Source: CAD feature listing. Evaluate the final solid. Frame: model axes, mm. Give positions to 0.01 mm unless a question says otherwise; leave off trailing zeros. Loops run counter-clockwise (first coordinate to the right, second up) from the corner with the lowest first, then second, coordinate; pieces in that order, holes last. Notation, with made-up numbers: M 14.25,13.25 L 55.25,13.25 A36 ccw 55.25,50.25 Z; hole C 3,72 d2. An arc over 180 degrees is marked long. Answer in a Markdown table with one row per item.
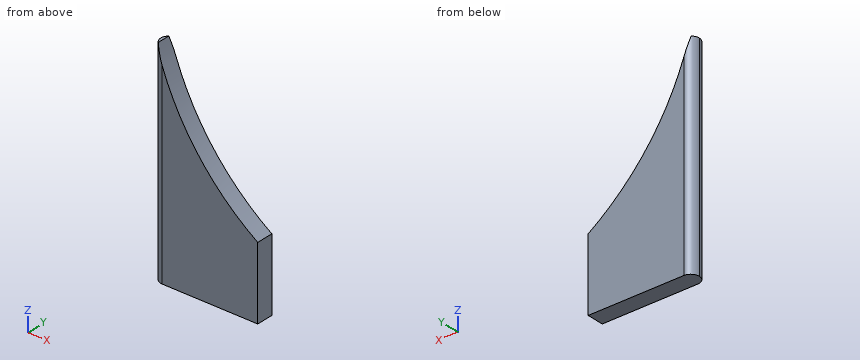
```python
from build123d import *

# Parameters (mm, degrees)
F1_DEPTH = 12
F2_R     = 5.99999


# Not quite as in the source:
# - a fillet or chamfer is up to 0.001 mm smaller than in the source, because OpenCascade refuses the exact size


with BuildPart() as f1:
    # F0 (on Front) → F1 (new body)
    with BuildSketch(Plane.XZ):
        with BuildLine():
            Line((-118, -20.6604213454), (-44.4413209303, -20.6604213454))
            Line((-44.4413209303, -20.6604213454), (-44.4413209303, 30.7246802683))
            ThreePointArc((-44.4413209303, 30.7246802683), (-89.0802193772, 73.6033003164), (-116, 129.3395786546))
            Line((-116, 129.3395786546), (-118, 129.3395786546))
            Line((-118, 129.3395786546), (-118, -20.6604213454))
        make_face()
    extrude(amount=F1_DEPTH)

    # F2 (radius 6 in the source; OpenCascade refuses exactly that, so slightly less here)
    f2_edges = [f1.edges().sort_by_distance(p)[0] for p in [
        (-118, 0, 54.339579),
        (-118, -12, 54.339579),
    ]]
    fillet(f2_edges, radius=F2_R)


solid = f1.part
```
Q1. Section query B-B (y = -8.5). Output: boundary loops of the cut face in (x, z).
Values follow:
| item | result |
|---|---|
| outline | M -117.45,-20.66 L -44.44,-20.66 L -44.44,30.72 A175 cw -116,129.34 L -117.45,129.34 Z |
Q2. Ray query, probe 1 along X at (y, z) = (-5.5, 29); probe 2 along X at (y, z) = (-8.25, -6.5); probe 3 along Z at (x, y) = (-94, -1). Return the intervals inside material, ascending. Write a range as from..to.
Values follow:
| item | result |
|---|---|
| probe 1 | -117.98..-44.44 |
| probe 2 | -117.56..-44.44 |
| probe 3 | -20.66..80.75 |
Q3. Section query C-C (x = -70.5). Output: boundary loops of the cut face in (y, z), plus the area to 3 significant figures.
Values follow:
| item | result |
|---|---|
| outline | M -12,-20.66 L 0,-20.66 L 0,51.96 L -12,51.96 Z |
| area | 871 mm^2 |
Q4. Contact query for a flat-ended pin moving along its axis: pin 1 Ø3 at (y, z) = (-8, 33.5) entering from +X. Output: stop coordinate, or through.
Values follow:
| item | result |
|---|---|
| pin 1 | x = -46.33 |
